from build123d import *

# Parameters (mm, degrees)
F0_R      = 24.3051606916
F1_DEPTH  = 5.08
F2_R      = 24.3051606916
F2_R_2    = 21.5505163445
F5_DEPTH  = 2.286
F4_R      = 21.5505163445
F4_R_2    = 17.3332692352
F6_DEPTH  = 1.778
F3_R      = 6.0083606655
F7_DEPTH  = 1.27
F8_R      = 1.4809931101
F9_DEPTH  = 2.54
F10_R     = 2.7483891527
F11_DEPTH = 25.4
F12_DEPTH = 27.94


with BuildPart() as f1:
    # F0 (on Front) → F1 (new body)
    with BuildSketch(Plane.XZ):
        Circle(F0_R)
    extrude(amount=F1_DEPTH)

    # F2 (on face) → F5 (join)
    with BuildSketch(Plane.XZ.offset(5.08)):
        Circle(F2_R)
        Circle(F2_R_2, mode=Mode.SUBTRACT)
    extrude(amount=F5_DEPTH)

    # F4 (on face) → F6 (join)
    with BuildSketch(Plane.XZ.offset(5.08)):
        Circle(F4_R)
        Circle(F4_R_2, mode=Mode.SUBTRACT)
    extrude(amount=F6_DEPTH)

    # F3 (on face) → F7 (join)
    with BuildSketch(Plane.XZ.offset(5.08)):
        Circle(F3_R)
    extrude(amount=F7_DEPTH)

    # F8 (on face) → F9 (join)
    with BuildSketch(Plane.XZ.offset(6.35)):
        Circle(F8_R)
    extrude(amount=F9_DEPTH)

    # F10 (on face) → F11 (cut)
    with BuildSketch(Plane.XZ.offset(5.08)):
        with Locations((0, 10.771388188)):
            Circle(F10_R)
        with Locations((7.6165216305, 7.6165216305)):
            Circle(F10_R)
        with Locations((10.771388188, 0)):
            Circle(F10_R)
        with Locations((7.6165216305, -7.6165216305)):
            Circle(F10_R)
        with Locations((0, -10.771388188)):
            Circle(F10_R)
        with Locations((-7.6165216305, -7.6165216305)):
            Circle(F10_R)
        with Locations((-10.771388188, 0)):
            Circle(F10_R)
        with Locations((-7.6165216305, 7.6165216305)):
            Circle(F10_R)
    extrude(amount=-F11_DEPTH, mode=Mode.SUBTRACT)

    # F12 (add): faces of the model
    f12_faces = [f1.faces().sort_by_distance(p)[0] for p in [
        (-20.9409756947, -6.858, 0),
        (-23.6177069339, -7.366, 0),
    ]]
    extrude(f12_faces, amount=F12_DEPTH)


solid = f1.part
The model under review builds one solid part; all positions refer to its coordinate system, in mm. A direction names the side the tool comes from. Round coordinates to 2 decimals unless told otherwise and drop trailing zeros. Order: outer loops, then holes, each group sorted by start corner. A loop starts at its lowest first (then second) coordinate and runs counter-clockwise, first axis right, second up. Notation, with made-up numbers: (-20.5, 33.25) - (-10.5, 33.25) arc R22 ccw to (-10.5, 52.25) - close; hole circle Ø4 at (-4.5, -18). An arc over 180 degrees is marked (long way). Use one line per item in the form item = value.
Q1. Add section D-D on y = -24. Give the boundary of the cut face in (x, z), then the cut area to 3 significant figures.
Response values:
outline = circle Ø48.61 at (0, 0); hole circle Ø34.67 at (0, 0)
area = 912 mm^2
Q2. Add section A-A on z = 0. Give the boundary of the cut face in (x, y), then the cut area to 3 significant figures.
Response values:
outline = (-24.31, -35.31) - (-21.55, -35.31) - (-21.55, -34.8) - (-17.33, -34.8) - (-17.33, -5.08) - (-13.52, -5.08) - (-13.52, 0) - (-24.31, 0) - close; (-8.02, -5.08) - (-6.01, -5.08) - (-6.01, -6.35) - (-1.48, -6.35) - (-1.48, -8.89) - (1.48, -8.89) - (1.48, -6.35) - (6.01, -6.35) - (6.01, -5.08) - (8.02, -5.08) - (8.02, 0) - (-8.02, 0) - close; (13.52, -5.08) - (17.33, -5.08) - (17.33, -34.8) - (21.55, -34.8) - (21.55, -35.31) - (24.31, -35.31) - (24.31, 0) - (13.52, 0) - close
area = 631 mm^2
Q3. Add section C-C on y = -4. Give the number of separate pieces and of enclosed holes in the cut face, then the cut area to 3 significant figures.
Response values:
separate_pieces = 1
enclosed_holes = 8
area = 1,670 mm^2
Q4. Mouldability with a two-part tool opening along Z and no side actions: class faces 1 (the flat face through (-15, -35.306, -16)), 2 (the cylindrical face through (-24.28, -17.41, 1.07)), 3 (the cylindrical face through (-0.596, -2.576, -13.454)), 4 (the flat face through (1, -34.798, 18)) as pulls with the +Z half, pulls with the -Z half, needs draft (parallel to the pull), parting line crosses it, or undercut.
Response values:
face_1 = needs draft
face_2 = parting line crosses it
face_3 = undercut
face_4 = undercut
Q5. Tool access review of faces 5 (the flat face through (0, 0, 0)), 6 (the cylindrical face through (1.413, -7.602, 0.445)): name each direction out of +Z, -Z, +X, -X, +Y, -Y from which nothing blocks a thin tool from reaching the whole face with its end or side.
Response values:
face_5 = +Z, -Z, +X, -X, +Y
face_6 = -Y
Q6. Clearance check with flat-ended pins moving along their axes: P1, Ø4.5, axis at x = 7.62, z = 7.62, coming from the -Y side; P2, Ø13, axis at x = 2, z = 0, coming from the -Y side; P3, Ø6.5, axis at x = -10.77, z = 0, coming from the -Y side; P4, Ø1, axis at x = -3, y = -8, coming from the +Z side. State where each tip first meets the part, or that it passes through.
Response values:
P1 = through
P2 = -8.89
P3 = -5.08
P4 = 24.18
Q7. Add section B-B on x = 0. Give the boundary of the cut face in (y, z).
Response values:
outline = (-35.31, -24.31) - (0, -24.31) - (0, -13.52) - (-5.08, -13.52) - (-5.08, -17.33) - (-34.8, -17.33) - (-34.8, -21.55) - (-35.31, -21.55) - close; (-35.31, 21.55) - (-34.8, 21.55) - (-34.8, 17.33) - (-5.08, 17.33) - (-5.08, 13.52) - (0, 13.52) - (0, 24.31) - (-35.31, 24.31) - close; (-8.89, -1.48) - (-6.35, -1.48) - (-6.35, -6.01) - (-5.08, -6.01) - (-5.08, -8.02) - (0, -8.02) - (0, 8.02) - (-5.08, 8.02) - (-5.08, 6.01) - (-6.35, 6.01) - (-6.35, 1.48) - (-8.89, 1.48) - close
Q8. To check wall thickness, follow line 1 (Z direction, x = 0, y = -35); line 2 (Y direction, x = 2.5, z = -6); line 3 (X direction, y = -10.5, z = -5). State the ranges of each line that lie inside material, in increasing order.
Response values:
line_1 = -24.31 to -21.55, 21.55 to 24.31
line_2 = -5.08 to 0
line_3 = -23.79 to -16.6, 16.6 to 23.79
